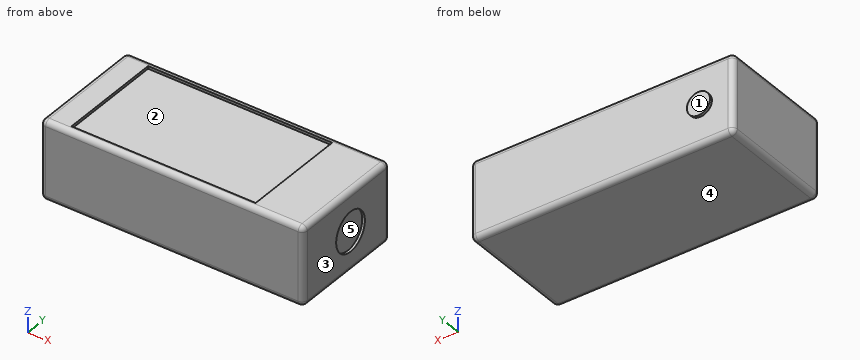
Autodesk Inventor part; units mm, degrees
ref_plane "YZ Plane" through (0, 0, 0) normal (1, 0, 0) x (0, 1, 0)
ref_plane "XZ Plane" through (0, 0, 0) normal (0, 1, 0) x (-1, 0, 0)
ref_plane "XY Plane" through (0, 0, 0) normal (0, 0, 1) x (1, 0, 0)
sketch "스케치1" plane through (0, 0, 0) normal (0, 0, 1) x (1, 0, 0)
  line L0 (0, 0) -> (100, 0)
  line L1 (100, 0) -> (100, 45)
  line L2 (100, 45) -> (0, 45)
  line L3 (0, 45) -> (0, 0)
  dimension "d0" = 100
  dimension "d1" = 45
extrude "돌출1" add sketch "스케치1" along normal mid plane 30
sketch "스케치2" plane through (100, 0, 15) normal (1, 0, 0) x (0, 0, -1)
  circle A0 centre (15, 24.5901) radius 7.5
  point P0 (15, 0)
  dimension "d4" = 15
extrude "돌출2" cut sketch "스케치2" against normal blind 1
sketch "스케치3" plane through (0, 0, 15) normal (0, 0, 1) x (1, 0, 0)
  line L0 (10, 42.5) -> (80, 42.5)
  line L1 (80, 42.5) -> (80, 2.5)
  line L2 (80, 2.5) -> (10, 2.5)
  line L3 (10, 2.5) -> (10, 42.5)
  line L4 (100, 45) -> (0, 45)
  line L5 (0, 45) -> (0, 0)
  dimension "d7" = 70
  dimension "d8" = 40
  dimension "d9" = 2.5
  dimension "d10" = 10
extrude "돌출3" cut sketch "스케치3" against normal blind 1
sketch "스케치4" plane through (0, 0, 14) normal (0, 0, 1) x (1, 0, 0)
  line L0 (11.7603, 30.0874) -> (53.0164, 30.0874) construction
  line L1 (53.0164, 30.0874) -> (53.0164, 23.3337) construction
  line L2 (53.0164, 23.3337) -> (11.7603, 23.3337) construction
  line L3 (11.7603, 23.3337) -> (11.7603, 30.0874) construction
  point P0 (0, 0)
sketch "스케치5" plane through (99, 24.5901, 0) normal (1, 0, 0) x (0, 0, -1)
  line L0 (-5.91, 1.6766) -> (6.6648, 1.6766) construction
  line L1 (6.6648, 1.6766) -> (6.6648, -1.7518) construction
  line L2 (6.6648, -1.7518) -> (-5.91, -1.7518) construction
  line L3 (-5.91, -1.7518) -> (-5.91, 1.6766) construction
  point P0 (0, -24.5901)
sketch "스케치6" plane through (0, 45, 15) normal (0, 1, 0) x (1, 0, 0)
  circle A0 centre (12.5978, 15) radius 4.3939
  point P0 (0, 15)
extrude "돌출4" add sketch "스케치6" along normal blind 1
sketch "스케치7" plane through (12.5978, 46, 0) normal (0, 1, 0) x (1, 0, 0)
  line L0 (-4.0633, 1.8765) -> (4.3199, 1.8765) construction
  line L1 (4.3199, 1.8765) -> (4.3199, -1.5495) construction
  line L2 (4.3199, -1.5495) -> (-4.0633, -1.5495) construction
  line L3 (-4.0633, -1.5495) -> (-4.0633, 1.8765) construction
  point P0 (-12.5978, 0)
fillet "모깎기1" radius 2 11 edges at (50, 45, 15) (100, 45, 0) (100, 22.5, 15) (100, 22.5, -15) (50, 45, -15) (50, 0, -15) (50, 0, 15) (100, 0, 0) (0, 0, 0) (0, 22.5, 15) (0, 22.5, -15)
fillet "모깎기2" radius 2 3 edges at (0, 45, 0) (0.5858, 44.4142, 14.4142) (0.5858, 44.4142, -14.4142)
properties part number "구상도"
Build history of the part. All positions in model axes, mm. Face numbers are marked on the shaded views. A direction names the side the tool comes from. Coordinates: 2 decimals unless noted, no trailing zeros. Order: outer loops, then holes, each group sorted by start corner. A loop starts at its lowest first (then second) coordinate and runs counter-clockwise, first axis right, second up. Notation, with made-up numbers: M 8.25,-30.75 L 38.25,-30.75 A29 cw 38.25,2.25 Z; hole C 11,15.25 d11. An arc over 180 degrees is marked long. One line per question, with ' | ' between items. Start each with the question number.
1. Tool access for the marked faces 4 and 5: list every direction of +Z, -Z, +X, -X, +Y, -Y with a clear straight run to the whole face (end or side of a thin tool).
2. Cut at B-B (y = 7). Write the cut outline in (x, z), plus the area to 3 significant figures.
3. Cut at D-D (z = 0). Write the cut outline in (x, y).
4. Flat gauge pins, fed straight in: P1, Ø12, axis at y = 38, z = -5, coming from the -X side; P2, Ø1.1, axis at x = 37.5, z = 14.5, coming from the -Y side; P3, Ø1.1, axis at y = 20, z = 14.5, coming from the -X side; P4, Ø4, axis at x = 40, z = -7, coming from the +Y side. Where does each tip first touch, or does it go through?
5. Wall check: line 1 along Y through (x, z) = (19.5, -13); line 2 along Z through (x, y) = (71.5, 8); line 3 along Y through (x, z) = (99.4, 0). Give the ranges that are in metal, low to high. Write a range as [from, to].
6. Cut at C-C (x = 56.5). Write the cut outline in (y, z), plus the area to 3 significant figures.
7. Cut at A-A (z = 10). Write the cut outline in (x, y).
8. Mould opens along X. For the marked faces 1, 2 and 3 say: +X half, -X half, draft (parallel to the pull), parting line (faces both ways), or undercut.
The answers:
1) face 4: -Z, +X, -X, +Y, -Y | face 5: +X
2) outline: M 0,-13 A2 ccw 2,-15 L 98,-15 A2 ccw 100,-13 L 100,13 A2 ccw 98,15 L 80,15 L 80,14 L 10,14 L 10,15 L 2,15 A2 ccw 0,13 Z | area: 2,930 mm2
3) outline: M 0,2 A2 ccw 2,0 L 98,0 A2 ccw 100,2 L 100,17.09 L 99,17.09 L 99,32.09 L 100,32.09 L 100,43 A2 ccw 98,45 L 16.99,45 L 16.99,46 L 8.2,46 L 8.2,45 L 2,45 A2 ccw 0,43 Z
4) P1: stops at x = 0 | P2: stops at y = 0.24 | P3: stops at x = 0.24 | P4: stops at y = 45
5) line 1: y = [0, 45] | line 2: z = [-15, 14] | line 3: y = [0.57, 17.09], [32.09, 44.43]
6) outline: M 0,-13 A2 ccw 2,-15 L 43,-15 A2 ccw 45,-13 L 45,13 A2 ccw 43,15 L 42.5,15 L 42.5,14 L 2.5,14 L 2.5,15 L 2,15 A2 ccw 0,13 Z | area: 1,310 mm2
7) outline: M 0,2 A2 ccw 2,0 L 98,0 A2 ccw 100,2 L 100,43 A2 ccw 98,45 L 2,45 A2 ccw 0,43 Z
8) face 1: draft | face 2: undercut | face 3: +X half
